Read the model definition and answer for the solid it produces. Units are mm, in the model's axes. Face numbers are marked on the shaded views. Give positions to 0.01 mm unless a question says otherwise; leave off trailing zeros. Order: outer loops, then holes, each group sorted by start corner. A loop starts at its lowest first (then second) coordinate and runs counter-clockwise, first axis right, second up. Notation, with made-up numbers: (35, 59.25) - (52, 59.25) arc R6 ccw to (52, 63.25) - close; hole circle Ø5 at (74, 76). An arc over 180 degrees is marked (long way). Write each question's results on one line, items separated by ' | '. Start each with the question number.
Q1. Find the intervals of material crossed by line 1 along X through (y, z) = (2, 0); line 2 along X through (y, z) = (0.9, -19.5); line 3 along Z through (x, y) = (-2, 5.75), in increasing order. Write a range as from..to.
Q2. Flat-ended cylindrical pins translate along their axes: P1, Ø6.5, axis at x = 0, z = -19.5, coming from the +Y side; P2, Ø3, axis at x = 4.5, y = 4.5, coming from the -Z side; P3, Ø1.5, axis at y = 5, z = -14, coming from the -X side. Find the tip coordinate at first contact, or state that the pin passes through.
Q3. For a pull along Z with two mould halves and no side action, classify the marked faces 1, 2 and 3 as +Z half, -Z half, draft (parallel to the pull), parting line (faces both ways), or undercut.
Q4. Find section C-C on z = 9.75. Give the vertices of the cut face in (x, y), and give its area (3 significant figures).
Q5. Find section A-A on x = 0. Give the vertices of the cut face in (y, z), and give its area (3 significant figures).
Q6. Find section B-B on z = 3. Give the vertices of the cut face in (x, y), and give its area (3 significant figures).
Q7. Find section D-D on y = 2. Give the vertices of the cut face in (x, z).
from build123d import *

# Parameters (mm, degrees)
SKETCH1_R                     = 25
SKETCH1_R_2                   = 10.5
BOSS_EXTRUDE1_DEPTH           = 6.5
CSK_FOR_M5_SFHCS1_D           = 5.5
CSK_FOR_M5_SFHCS1_CSINK_D     = 11.2
CSK_FOR_M5_SFHCS1_CSINK_ANGLE = 90
CIRPATTERN1_COUNT             = 3


with BuildPart() as part:
    # Sketch1 → Boss-Extrude1 (new body)
    with BuildSketch(Plane(origin=(0, 0, 0), x_dir=(1, 0, 0), z_dir=(0, 1, 0))):
        with Locations(Location((0, 0, 0), (0, 0, 90))):
            Circle(SKETCH1_R)
        with Locations(Location((0, 0, 0), (0, 0, 90))):
            Circle(SKETCH1_R_2, mode=Mode.SUBTRACT)
    extrude(amount=BOSS_EXTRUDE1_DEPTH)

    # CSK for M5 SFHCS1 (through all)
    with Locations(Plane(origin=(0, 6.5, 0), x_dir=(1, 0, 0), z_dir=(0, 1, 0))):
        with Locations((0, 19.5)):
            csk_for_m5_sfhcs1 = CounterSinkHole(CSK_FOR_M5_SFHCS1_D / 2, CSK_FOR_M5_SFHCS1_CSINK_D / 2, counter_sink_angle=CSK_FOR_M5_SFHCS1_CSINK_ANGLE)

    # CirPattern1: CSK for M5 SFHCS1 ×3 about axis
    cirpattern1_axis = Axis((0, 0, 0), (0, 1, 0))
    for i in range(1, CIRPATTERN1_COUNT):
        add(csk_for_m5_sfhcs1.rotate(cirpattern1_axis, i * 360 / CIRPATTERN1_COUNT), mode=Mode.SUBTRACT)


solid = part.part
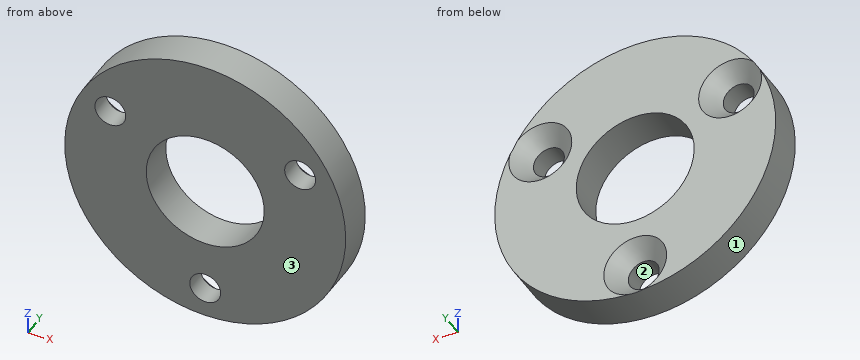
Working result:
1) line 1: -25..-10.5, 10.5..25 | line 2: -15.64..-2.75, 2.75..15.64 | line 3: -24.92..-23.92, -15.08..-10.31, 10.31..24.92
2) P1: y = 4.15 | P2: z = -24.82 | P3: x = -21.2
3) face 1: parting line | face 2: undercut | face 3: draft
4) outline: (-23.02, 0) - (-19.64, 0) - (-19.64, 3.65) - (-22.49, 6.5) - (-23.02, 6.5) - close; (-14.14, 0) - (-3.9, 0) - (-3.9, 6.5) - (-11.29, 6.5) - (-14.14, 3.65) - close; (3.9, 0) - (14.14, 0) - (14.14, 3.65) - (11.29, 6.5) - (3.9, 6.5) - close; (19.64, 0) - (23.02, 0) - (23.02, 6.5) - (22.49, 6.5) - (19.64, 3.65) - close | area: 161 mm²
5) outline: (0, -25) - (6.4, -25) - (3.65, -22.25) - (0, -22.25) - close; (0, -16.75) - (3.65, -16.75) - (6.5, -13.9) - (6.5, -10.5) - (0, -10.5) - close; (0, 10.5) - (6.5, 10.5) - (6.5, 25) - (0, 25) - close | area: 145 mm²
6) outline: (-24.82, 0) - (-10.06, 0) - (-10.06, 6.5) - (-24.82, 6.5) - close; (10.06, 0) - (24.82, 0) - (24.82, 6.5) - (10.06, 6.5) - close | area: 192 mm²
7) outline: circle Ø50 at (0, 0); hole circle Ø5.5 at (-16.89, 9.75); hole circle Ø21 at (0, 0); hole circle Ø5.5 at (0, -19.5); hole circle Ø5.5 at (16.89, 9.75)
